from build123d import *

# Parameters (mm, degrees)
F1_DEPTH = 8
F2_R     = 2
F3_R     = 1
F4_R     = 2
F5_R     = 0.99999


# Not quite as in the source:
# - a fillet or chamfer is up to 0.001 mm smaller than in the source, because OpenCascade refuses the exact size


with BuildPart() as f1:
    # F0 (on Top) → F1 (new body)
    with BuildSketch(Plane.XY):
        with BuildLine():
            Line((20, 0), (0, 0))
            Line((0, 0), (0, -2))
            Line((0, -2), (23, -2))
            Line((23, -2), (23, 4.5))
            Line((23, 4.5), (0, 4.5))
            Line((0, 4.5), (0, 3.478939205))
            ThreePointArc((0, 3.478939205), (-0.3538557851, 1.6956316782), (1.2766015908, 2.5))
            Line((1.2766015908, 2.5), (20, 2.5))
            Line((20, 2.5), (20, 0))
        make_face()
    extrude(amount=F1_DEPTH)

    # F2
    f2_edges = [f1.edges().sort_by_distance(p)[0] for p in [
        (23, -2, 4),
        (23, 4.5, 4),
        (0, 3.478939, 4),
    ]]
    fillet(f2_edges, radius=F2_R)

    # F3
    f3_edges = [f1.edges().sort_by_distance(p)[0] for p in [
        (1.276602, 2.5, 4),
    ]]
    fillet(f3_edges, radius=F3_R)

    # F4
    f4_edges = [f1.edges().sort_by_distance(p)[0] for p in [
        (0, 4.5, 4),
    ]]
    fillet(f4_edges, radius=F4_R)

    # F5 (radius 1 in the source; OpenCascade refuses exactly that, so slightly less here)
    f5_edges = [f1.edges().sort_by_distance(p)[0] for p in [
        (0, 0, 4),
        (0, -2, 4),
    ]]
    fillet(f5_edges, radius=F5_R)


solid = f1.part
Read the model definition and answer for the solid it produces. Units are mm, in the model's axes. A direction names the side the tool comes from. Round coordinates to 2 decimals unless told otherwise and drop trailing zeros. Loops run counter-clockwise (first coordinate to the right, second up) from the corner with the lowest first, then second, coordinate; pieces in that order, holes last.
Q1. Section B-B on y = 1.25 is taken. Write down the section's boundary in (x, z), and give its area (3 significant figures).
Q2. Determine the mould class of faces 1 (the face through (20, 1, 4)), 2 (the face through (0.301, -1.715, 4.056)), 3 (the face through (11, 3, 0)) for opening direction Y: released by +Y, released by -Y, zero draft, split by the parting line, or undercut.
Q3. Section C-C on x = 21.5 is taken. Write down the section's boundary in (y, z), and give its area (3 significant figures).
Q4. Section A-A on x = 8 is taken. Write down the section's boundary in (y, z).
Q5. Consider probe 1 along Y at (x, z) = (6, 4.5); probe 2 along X at (y, z) = (2, 3.5); probe 3 along Y at (x, z) = (1.5, 6). Determine where each line is inside the solid, lowest interval first.
Q6. This flat-tipped pin is pushed along its axis until it touches: pin 1 (2 mm diameter, centred on y = 1, z = 2, fed in from -X). Where does it stop, or does it pass through?
Q7. Which of the six approach directions +Z, -Z, +X, -X, +Y, -Y give full straight-line access (tool end or side, diameter ignored) to faces 4 (the face through (22.4, -1.43, 4.06)), 5 (the face through (11, 2.5, 4)), 6 (the face through (0.301, -0.285, 4.056))?
Output:
1. outline: (20, 0) - (23, 0) - (23, 8) - (20, 8) - close
1. area: 24.0 mm2
2. face 1: undercut
2. face 2: released by -Y
2. face 3: zero draft
3. outline: (-1.94, 0) - (4.44, 0) - (4.44, 8) - (-1.94, 8) - close
3. area: 51.0 mm2
4. outline: (-2, 0) - (0, 0) - (0, 8) - (-2, 8) - close; (2.5, 0) - (4.5, 0) - (4.5, 8) - (2.5, 8) - close
5. probe 1: y = -2 to 0, 2.5 to 4.5
5. probe 2: x = -0.62 to 1.14, 20 to 23
5. probe 3: y = -2 to 0, 2.36 to 4.5
6. pin 1: stops at x = -0.62
7. face 4: +Z, -Z, +X, -Y
7. face 5: +Z, -Z
7. face 6: +Z, -Z, -X
